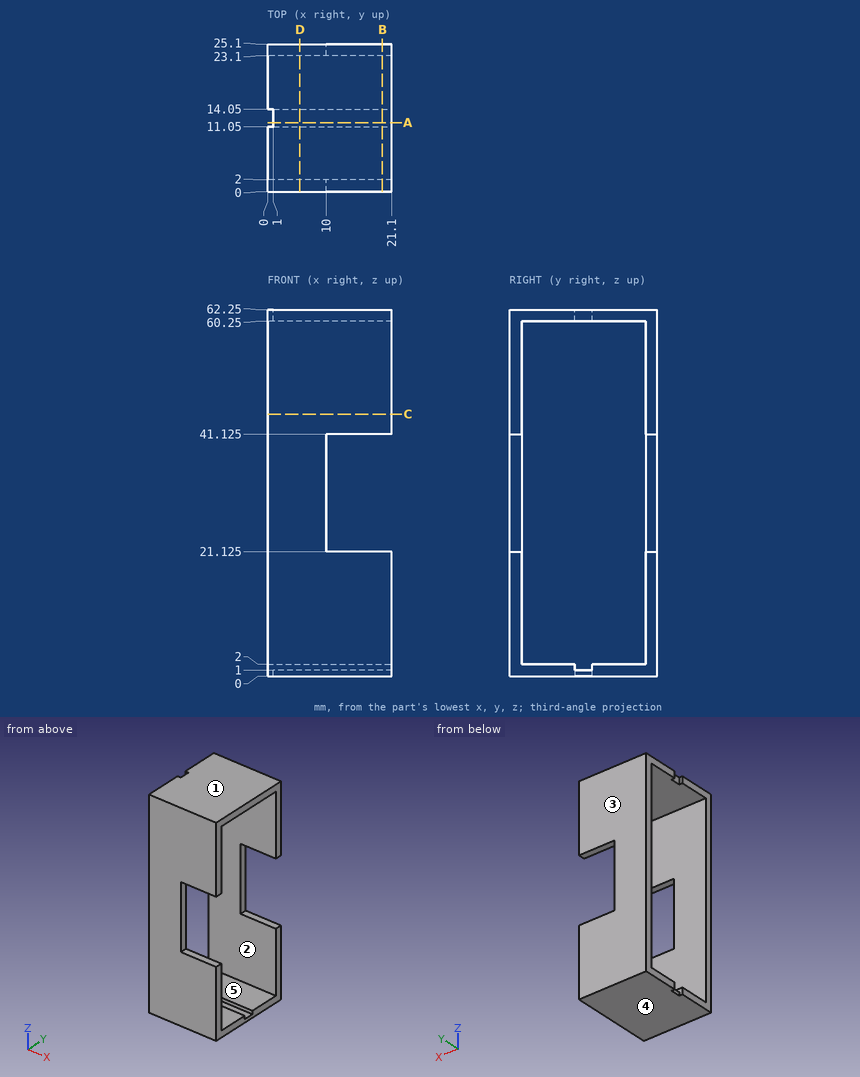
Can you work these out from the drawing? Everything is in mm from the part's minimum corner. A direction names the side the tool comes from. Round coordinates to 2 decimals unless told otherwise and drop trailing zeros. Order: outer loops, then holes, each group sorted by start corner. A loop starts at its lowest first (then second) coordinate and runs counter-clockwise, first axis right, second up. Notation, with made-up numbers: M 77.5,75.5 L 88.5,75.5 A18 ccw 88.5,101.5 Z; hole C 42,58.5 d1. An arc over 180 degrees is marked long. One line per question, with ' | ' between items.
1) I want a section at B-B, the plane x = 19.5. Write out the boundary of the cut face in (y, z) (3 decimals).
Working result:
outline: M 0,0 L 25.1,0 L 25.1,21.125 L 23.1,21.125 L 23.1,2 L 14.05,2 L 14.05,1 L 11.05,1 L 11.05,2 L 2,2 L 2,21.125 L 0,21.125 Z; M 0,41.125 L 2,41.125 L 2,60.25 L 23.1,60.25 L 23.1,41.125 L 25.1,41.125 L 25.1,62.25 L 0,62.25 Z
2) I need wall thicknesses on line 1 along Y through (x, z) = (10, 10); line 2 along Z through (x, y) = (5.5, 7.5); line 3 along Z through (x, y) = (6, 12.5). Which ranges of each line are inside material? Lowest first, please.
Working result:
line 1: 0 to 2, 23.1 to 25.1 | line 2: 0 to 2, 60.25 to 62.25 | line 3: 0 to 1, 60.25 to 62.25
3) I want a section at D-D, the plane x = 5.5. Write out the boundary of the cut face in (y, z).
Working result:
outline: M 0,0 L 25.1,0 L 25.1,62.25 L 0,62.25 Z; hole M 2,2 L 11.05,2 L 11.05,1 L 14.05,1 L 14.05,2 L 23.1,2 L 23.1,60.25 L 2,60.25 Z
4) For the marked faces 1 and 2, which set-ups out of +Z, -Z, +X, -X, +Y, -Y let a thin tool reach every point of the face, with its end or its side?
Working result:
face 1: +Z, +X, -X, +Y, -Y | face 2: +X, -X
5) For pin 1 Ø1 at (y, z) = (24, 31.5) entering from +X; pin 2 Ø0.5 at (y, z) = (12.5, 0.5) entering from -X, each with a flat end and sliding along its axis, tell me the tip position at first contact or that it passes through.
Working result:
pin 1: x = 10 | pin 2: x = 1
6) I want a section at C-C, the plane z = 44.5. Write out the boundary of the cut face in (x, y), then the cut area to 3 significant figures.
Working result:
outline: M 0,0 L 21.1,0 L 21.1,2 L 0,2 Z; M 0,23.1 L 21.1,23.1 L 21.1,25.1 L 0,25.1 Z | area: 84.4 mm²
7) I want a section at A-A, the plane y = 11.75. Write out the boundary of the cut face in (x, z).
Working result:
outline: M 1,0 L 21.1,0 L 21.1,1 L 1,1 Z; M 1,60.25 L 21.1,60.25 L 21.1,62.25 L 1,62.25 Z
8) If we mould it in two halves opening along Z, with no side actions, what happens to the marked faces 3, 4 and 5? For each: +Z half, -Z half, draft (parallel to the pull), parting line (faces both ways), or undercut.
Working result:
face 3: draft | face 4: -Z half | face 5: undercut
